For this review, take the finished solid that the model builds, in its own axes (mm). A direction names the side the tool comes from. Coordinates: 2 decimals unless noted, no trailing zeros. Loops run counter-clockwise (first coordinate to the right, second up) from the corner with the lowest first, then second, coordinate; pieces in that order, holes last. Notation, with made-up numbers: (-20.5, -27) - (24.5, -27) arc R33 cw to (24.5, 8) - close; hole circle Ø2 at (-30, 69.25). An arc over 180 degrees is marked (long way). Use one line per item in the form item = value. Start each with the question number.
1. Draft analysis for pull direction Y (two halves, no side actions). For faces 4 (the face through (-2.66, -1.08, -4.88)), 5 (the face through (-6, 2, -2)), 6 (the face through (-4.521, 2.155, -1.267)), 7 (the face through (-4.521, -2.155, 1.267)), state which applies: +Y half, -Y half, draft (parallel to the pull), parting line (faces both ways), or undercut.
2. For pin 1 Ø1 at (y, z) = (-3.5, 4) entering from -X; pin 2 Ø3 at (x, y) = (-1, 3) entering from -Z; pin 3 Ø1.4 at (x, y) = (-4.5, -0.5) entering from -Z; pin 4 Ø0.9 at (y, z) = (1.5, 0.5) entering from -X, all flat-tipped, find the tip position at first contact; note any pin that passes through.
3. To check wall thickness, follow probe 1 along X at (y, z) = (3, 2.5); probe 2 along Z at (x, y) = (-5, -2.5); probe 3 along Z at (x, y) = (-4.25, 0.25). State the ranges of each line that lie inside material, in increasing order.
4. Add section A-A on x = 13. Give the boundary of the cut face in (y, z), and give its area (3 significant figures).
5. Machinability: for faces 1 (the face through (15, 0, 0)), 2 (the face through (0, 3.3, 0.1)), 3 (the face through (-5, 0, -2.5)), which of the approach directions +Z, -Z, +X, -X, +Y, -Y give a long, thin tool a straight path to every point of the face, cutting with its end or side? Answer none if there is none.
Autodesk Inventor part; units mm, degrees
ref_plane "to_cp_XY" through (0, 0, 0) normal (1, 0, 0) x (0, 0, -1)
ref_plane "to_cp_YZ" through (0, 0, 0) normal (0, 0, -1) x (0, 1, 0)
ref_plane "to_cp_ZX" through (0, 0, 0) normal (0, 1, 0) x (1, 0, 0)
sketch "Sketch_1" plane through (0, 0, 0) normal (0, 0, 1) x (1, 0, 0)
  line L0 (15, 0) -> (-6, 0)
  line L1 (-6, 0) -> (-6, 4.4)
  line L2 (-6, 4.4) -> (-5.4, 5)
  line L3 (-5.4, 5) -> (0, 5)
  line L4 (0, 5) -> (0, 3)
  line L5 (0, 3) -> (14.3865, 3)
  line L6 (14.3865, 3) -> (15, 2.3865)
  line L7 (15, 2.3865) -> (15, 0)
  line L8 (15, 0) -> (-6, 0)
revolve "Revolution1" add sketch "Sketch_1" angle 360 about axis through (15, 0, 0) along (1, 0, 0)
thread "Thread1"
sketch "Sketch2" plane through (-6, 0, 0) normal (-1, 0, 0) x (0, 0, 1)
  point P0 (0, 0)
hole "Hole1" at (-6, 0, 0) direction (1, 0, 0) diameter 5 depth 3 tip angle 150
sketch "Sketch_3" plane through (-6, 0, 0) normal (1, 0, 0) x (0, 0, -1)
  line L0 (-2.5, -1.4434) -> (0, -2.8868)
  line L1 (0, -2.8868) -> (2.5, -1.4434)
  line L2 (2.5, -1.4434) -> (2.5, 1.4434)
  line L3 (2.5, 1.4434) -> (0, 2.8868)
  line L4 (0, 2.8868) -> (-2.5, 1.4434)
  line L5 (-2.5, 1.4434) -> (-2.5, -1.4434)
extrude "Extrusion1" cut sketch "Sketch_3" along normal blind 3
ref_plane "to_cp_XY" through (0, 0, 0) normal (1, 0, 0) x (0, 0, -1)
ref_plane "to_cp_YZ" through (0, 0, 0) normal (0, 0, -1) x (0, 1, 0)
ref_plane "to_cp_ZX" through (0, 0, 0) normal (0, 1, 0) x (1, 0, 0)
properties part number "BOLT6-15"
Conclusion:
q1.face_4 = parting line
q1.face_5 = draft
q1.face_6 = undercut
q1.face_7 = undercut
q2.pin_1 = -5.58
q2.pin_2 = -4.77
q2.pin_3 = -5
q2.pin_4 = -2.87
q3.probe_1 = -6 to 0
q3.probe_2 = -4.33 to -0.67, 0.67 to 4.33
q3.probe_3 = -4.99 to -2.5, 2.5 to 4.99
q4.outline = circle Ø6 at (0, 0)
q4.area = 28.3 mm^2
q5.face_1 = +Z, -Z, +X, +Y, -Y
q5.face_2 = +X
q5.face_3 = -X
